For this review, take the finished solid that the model builds, in its own axes (mm). Face numbers are marked on the shaded views. A direction names the side the tool comes from. Round coordinates to 2 decimals unless told otherwise and drop trailing zeros. Order: outer loops, then holes, each group sorted by start corner. A loop starts at its lowest first (then second) coordinate and runs counter-clockwise, first axis right, second up. Notation, with made-up numbers: (0.5, 11.5) -> (49.5, 11.5) arc R28 cw to (49.5, 35.5) -> close; hole circle Ø6 at (-2, 89.25). An arc over 180 degrees is marked (long way). Use a Markdown table: item, result. Add a question column.
1) Machinability: for the marked faces 4 and 5, which of the approach directions +Z, -Z, +X, -X, +Y, -Y give a long, thin tool a straight path to every point of the face, cutting with its end or side? Answer none if there is none.
2) Draft analysis for pull direction Z (two halves, no side actions). For the marked faces 1, 2 and 3, state which applies: pulls with the +Z half, pulls with the -Z half, needs draft (parallel to the pull), parting line crosses it, or undercut.
3) Consider section D-D (x = 14). State the section outline as (y, z) points.
4) Clearance check with flat-ended pins moving along their axes: P1, Ø3, axis at x = -8, z = -8, coming from the +Y side; P2, Ø2, axis at x = -4.5, z = 11.5, coming from the -Y side; P3, Ø1.9, axis at x = 4, z = 12, coming from the -Y side. State where each tip first meets the part, or that it passes through.
5) Wall thickness on line 1 along X through (y, z) = (3.1, 4); line 2 along X through (y, z) = (0.8, 12); line 3 along X through (y, z) = (1.9, -11): over which ranges is each line inside the solid? List them lowest first. Write a range as [from, to].
6) Consider section A-A (y = 1.6). Give the number of separate pieces and of enclosed holes in the cut face, plus the area to 3 significant figures.
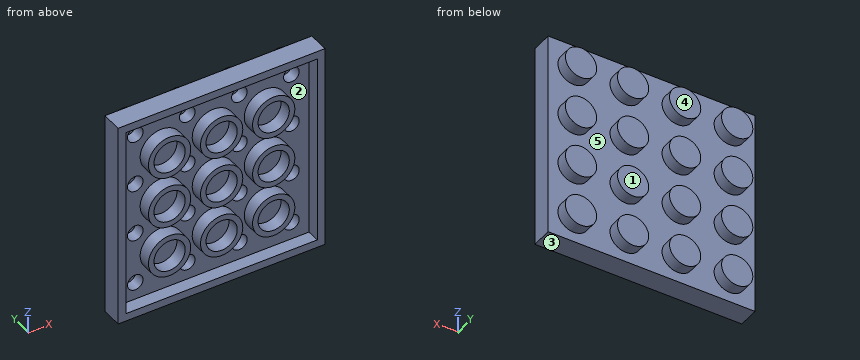
```python
from build123d import *

# Parameters (mm, degrees)
SKETCH1_W            = 31.8
SKETCH1_H            = 31.8
BOSS_EXTRUDE1_DEPTH  = 3.2
SKETCH2_R            = 2.4
BOSS_EXTRUDE2_DEPTH  = 1.8
LPATTERN1_COUNT      = 4
LPATTERN1_PITCH      = 8
LPATTERN1_COUNT_DIR2 = 4
LPATTERN1_PITCH_DIR2 = 8
SHELL1_T             = -1.2
SKETCH3_R            = 3.25
SKETCH3_R_2          = 2.4
BOSS_EXTRUDE3_DEPTH  = 2
LPATTERN2_COUNT      = 3
LPATTERN2_PITCH      = 8
LPATTERN2_COUNT_DIR2 = 3
LPATTERN2_PITCH_DIR2 = 8


with BuildPart() as part:
    # Sketch1 → Boss-Extrude1 (new body)
    with BuildSketch(Plane(origin=(0, 0, 0), x_dir=(1, 0, 0), z_dir=(0, 1, 0))):
        Rectangle(SKETCH1_W, SKETCH1_H)
    extrude(amount=BOSS_EXTRUDE1_DEPTH)

    # Sketch2 → Boss-Extrude2 (add)
    with BuildSketch(Plane(origin=(0, 3.2, 0), x_dir=(1, 0, 0), z_dir=(0, 1, 0))):
        with Locations(Location((-12, -12, 0), (0, 0, 90))):
            Circle(SKETCH2_R)
    boss_extrude2 = extrude(amount=BOSS_EXTRUDE2_DEPTH)

    # LPattern1: Boss-Extrude2 4 × 4
    with Locations(*[(i * LPATTERN1_PITCH, 0, -j * LPATTERN1_PITCH_DIR2) for i in range(LPATTERN1_COUNT) for j in range(LPATTERN1_COUNT_DIR2) if (i, j) != (0, 0)]):
        add(boss_extrude2)

    # Shell1
    shell1_openings = [part.faces().sort_by_distance(p)[0] for p in [
        (0, 0, 0),
    ]]
    offset(amount=SHELL1_T, openings=shell1_openings, kind=Kind.INTERSECTION)

    # Sketch3 → Boss-Extrude3 (add)
    with BuildSketch(Plane.XZ.offset(-2)):
        with Locations(Location((-8, 8, 0), (0, 0, 270))):
            Circle(SKETCH3_R)
        with Locations(Location((-8, 8, 0), (0, 0, 270))):
            Circle(SKETCH3_R_2, mode=Mode.SUBTRACT)
    boss_extrude3 = extrude(amount=BOSS_EXTRUDE3_DEPTH)

    # LPattern2: Boss-Extrude3 3 × 3
    with Locations(*[(i * LPATTERN2_PITCH, 0, -j * LPATTERN2_PITCH_DIR2) for i in range(LPATTERN2_COUNT) for j in range(LPATTERN2_COUNT_DIR2) if (i, j) != (0, 0)]):
        add(boss_extrude3)


solid = part.part
```
Results list:
| question | item | result |
|---|---|---|
| 1 | face 4 | +Z, -Z, +X, -X, +Y |
| 1 | face 5 | +Y |
| 2 | face 1 | needs draft |
| 2 | face 2 | undercut |
| 2 | face 3 | pulls with the -Z half |
| 3 | outline | (0, -15.9) -> (3.2, -15.9) -> (3.2, -13.33) -> (5, -13.33) -> (5, -10.67) -> (3.2, -10.67) -> (3.2, -5.33) -> (5, -5.33) -> (5, -2.67) -> (3.2, -2.67) -> (3.2, 2.67) -> (5, 2.67) -> (5, 5.33) -> (3.2, 5.33) -> (3.2, 10.67) -> (5, 10.67) -> (5, 13.33) -> (3.2, 13.33) -> (3.2, 15.9) -> (0, 15.9) -> (0, 14.7) -> (2, 14.7) -> (2, -14.7) -> (0, -14.7) -> close |
| 4 | P1 | y = 3.2 |
| 4 | P2 | y = 2 |
| 4 | P3 | y = 3.8 |
| 5 | line 1 | [-15.9, -13.2], [-10.8, -5.2], [-2.8, 2.8], [5.2, 10.8], [13.2, 15.9] |
| 5 | line 2 | [-15.9, -14.7], [14.7, 15.9] |
| 5 | line 3 | [-15.9, -14.7], [-9.25, -6.75], [-1.25, 1.25], [6.75, 9.25], [14.7, 15.9] |
| 6 | separate pieces | 10 |
| 6 | enclosed holes | 10 |
| 6 | area | 283 mm2 |
